```python
from build123d import *

# Parameters (mm, degrees)
SKETCH_1_W          = 19
SKETCH_1_H          = 15
SKETCH_1_R          = 1.1
EXTRUDE_1_DEPTH     = 1.5
SKETCH_1_4_R        = 2.4
EXTRUDE_2_DEPTH     = 14
SKETCH_1_5_R        = 2.85
EXTRUDE_3_DEPTH     = 5.86
SKETCH_1_7_R        = 2.85
CUT_EXTRUDE_1_DEPTH = 4.86
SKETCH_1_8_W        = 0.5
SKETCH_1_8_H        = 0.5
EXTRUDE_4_DEPTH     = 4.86
FILLET_3_SIZE       = 1.5
FILLET_3_SIZE_2     = 2
SKETCH_1_9_W        = 2.5
SKETCH_1_9_H        = 10
EXTRUDE_5_DEPTH     = 4.6


with BuildPart() as part:
    # Sketch 1 → Extrude 1 (new body)
    with BuildSketch(Plane(origin=(0, 0, 0), x_dir=(1, 0, 0), z_dir=(0, 1, 0))):
        with Locations((9.5, 7.5)):
            Rectangle(SKETCH_1_W, SKETCH_1_H)
        with Locations(Location((17, 13, 0), (0, 0, 270))):
            Circle(SKETCH_1_R, mode=Mode.SUBTRACT)
        with Locations(Location((17, 2, 0), (0, 0, 270))):
            Circle(SKETCH_1_R, mode=Mode.SUBTRACT)
    extrude(amount=-EXTRUDE_1_DEPTH)

    # Sketch 1_4 → Extrude 2 (add)
    with BuildSketch(Plane(origin=(0, 0, 0), x_dir=(1, 0, 0), z_dir=(0, 1, 0))):
        with Locations(Location((10, 7.5, 0), (0, 0, 270))):
            Circle(SKETCH_1_4_R)
    extrude(amount=EXTRUDE_2_DEPTH)

    # Sketch 1_5 → Extrude 3 (add)
    with BuildSketch(Plane(origin=(0, 0, 0), x_dir=(1, 0, 0), z_dir=(0, 1, 0))):
        with Locations(Location((10, 7.5, 0), (0, 0, 90))):
            Circle(SKETCH_1_5_R)
    extrude(amount=EXTRUDE_3_DEPTH)

    # Sketch 1_7 → Cut-Extrude 1 (cut)
    with BuildSketch(Plane(origin=(0, 0, 0), x_dir=(1, 0, 0), z_dir=(0, 1, 0))):
        with Locations(Location((10, 7.5, 0), (0, 0, 90))):
            Circle(SKETCH_1_7_R)
    extrude(amount=CUT_EXTRUDE_1_DEPTH, mode=Mode.SUBTRACT)


with BuildPart() as cut_extrude_1_piece_1:
    # of the separate pieces the step leaves, piece 1, a body of its own (cut_extrude_1_pieces)
    add(part.part.solids().sort_by_distance((0, 0, 0))[0])



with BuildPart() as cut_extrude_1_piece_2:
    # of the separate pieces the step leaves, piece 2, a body of its own (cut_extrude_1_pieces)
    add(part.part.solids().sort_by_distance((10, 4.86, -10.35))[0])


with BuildPart() as cut_extrude_1_piece_1_1:
    add(cut_extrude_1_piece_1.part)

    add(cut_extrude_1_piece_2.part)  # Extrude 4 merges Cut-Extrude 1 piece 2
    # Sketch 1_8 → Extrude 4 (add)
    with BuildSketch(Plane(origin=(0, 0, 0), x_dir=(1, 0, 0), z_dir=(0, 1, 0))):
        with Locations((9.262196887, 8.297981086)):
            Rectangle(SKETCH_1_8_W, SKETCH_1_8_H)
        with Locations((9.191679648, 6.064699679)):
            Rectangle(SKETCH_1_8_W, SKETCH_1_8_H)
        with Locations((10.845962172, 6.664377094)):
            Rectangle(SKETCH_1_8_W, SKETCH_1_8_H)
        with Locations((10.845962172, 8.732230249)):
            Rectangle(SKETCH_1_8_W, SKETCH_1_8_H)
    extrude(amount=EXTRUDE_4_DEPTH)

    # Fillet 3
    # an asymmetric fillet: 2, 1.5 mm, written as the material it takes off along each edge
    with BuildSketch(Plane(origin=(10, 14, -7.5), x_dir=(0, 0, 1), z_dir=(-1, 0, 0))) as fillet_3_piece_1:
        with BuildLine():
            Bezier((2.4, -FILLET_3_SIZE), (2.4, 0), (2.4 - FILLET_3_SIZE_2, 0), weights=[1, 0.707106781, 1])
            Line((2.4 - FILLET_3_SIZE_2, 0), (2.4, 0))
            Line((2.4, 0), (2.4, -FILLET_3_SIZE))
        make_face()
    revolve(axis=Axis((10, 14, -7.5), (0, 1, 0)), mode=Mode.SUBTRACT)

    # Sketch 1_9 → Extrude 5 (add)
    with BuildSketch(Plane(origin=(0, 0, 0), x_dir=(1, 0, 0), z_dir=(0, 1, 0))):
        with Locations((2.25, 7.5)):
            Rectangle(SKETCH_1_9_W, SKETCH_1_9_H)
    extrude(amount=EXTRUDE_5_DEPTH)


solid = cut_extrude_1_piece_1_1.part
```
Geometry check sheet. Reference: the model listing, model coordinates, mm. A direction names the side the tool comes from. Coordinates: 2 decimals unless noted, no trailing zeros. Order: outer loops, then holes, each group sorted by start corner. A loop starts at its lowest first (then second) coordinate and runs counter-clockwise, first axis right, second up. Notation, with made-up numbers: M -15,87 L -3,87 A23 cw -3,123 Z; hole C -37,-26.5 d4. An arc over 180 degrees is marked long. One line per question, with ' | ' between items. Start each with the question number.
Item 1: Cross-section at C-C on x = 17. Enter the section's corners in (y, z).
Item 2: Set-up check for faces 1 (the flat face through (2, 2, -2.5)), 2 (the flat face through (11, 5.86, -5)), 3 (the flat face through (2, 2, -12.5)): record each of +Z, -Z, +X, -X, +Y, -Y from which the full face is reachable in a straight line by a thin tool's end or side.
Item 3: Cross-section at B-B on z = -13. Enter the section's corners in (x, y), then the cut area to 3 significant figures.
Item 4: Cross-section at D-D on x = 3.25. Enter the section's corners in (y, z), then the cut area to 3 significant figures.
Item 5: Cross-section at A-A on y = 2.75. Enter the section's corners in (x, z).
Item 6: Draft check along X on faces 4 (the cylindrical face through (15.926, -0.74, -2.238)), 5 (the flat face through (19, -1, -7)), 6 (the flat face through (9, -1, 0)). Enter one of: pulls with the +X half, pulls with the -X half, needs draft (parallel to the pull), parting line crosses it, or undercut.
Item 7: Gauge pin test, flat ends, axial feed: pin 1 (2 mm diameter, centred on x = 17, z = -2, fed in from +Y) (3 decimals); pin 2 (2 mm diameter, centred on x = 6, z = -2.5, fed in from +Y); pin 3 (0.8 mm diameter, centred on x = 3, z = -6.5, fed in from +Y); pin 4 (0.6 mm diameter, centred on y = 3, z = -6.5, fed in from +X). Record the tip position at first contact, or that the pin passes through.
Item 8: Material ranges on L1, parallel to X at y = -1.1, z = -2; L2, parallel to Y at x = 3, z = -5; L3, parallel to Y at x = 7.25, z = -1, recorded low to high. Write a range as [from, to].
Findings:
1) outline: M -1.5,-15 L 0,-15 L 0,-14.1 L -1.5,-14.1 Z; M -1.5,-11.9 L 0,-11.9 L 0,-3.1 L -1.5,-3.1 Z; M -1.5,-0.9 L 0,-0.9 L 0,0 L -1.5,0 Z
2) face 1: +Z, +X, -X, +Y | face 2: +Y | face 3: -Z, +X, -X, +Y
3) outline: M 0,-1.5 L 15.9,-1.5 L 15.9,0 L 0,0 Z; M 18.1,-1.5 L 19,-1.5 L 19,0 L 18.1,0 Z | area: 25.2 mm²
4) outline: M -1.5,-15 L 0,-15 L 0,-12.5 L 4.6,-12.5 L 4.6,-2.5 L 0,-2.5 L 0,0 L -1.5,0 Z | area: 68.5 mm²
5) outline: M 1,-12.5 L 3.5,-12.5 L 3.5,-2.5 L 1,-2.5 Z; M 8.94,-6.31 L 9.44,-6.31 L 9.44,-5.81 L 8.94,-5.81 Z; M 9.01,-8.55 L 9.51,-8.55 L 9.51,-8.05 L 9.01,-8.05 Z; M 10.6,-8.98 L 11.1,-8.98 L 11.1,-8.48 L 10.6,-8.48 Z; M 10.6,-6.91 L 11.1,-6.91 L 11.1,-6.41 L 10.6,-6.41 Z
6) face 4: undercut | face 5: pulls with the +X half | face 6: needs draft
7) pin 1: passes through | pin 2: stops at y = 0 | pin 3: stops at y = 4.6 | pin 4: stops at x = 11.1
8) L1: x = [0, 15.9], [18.1, 19] | L2: y = [-1.5, 4.6] | L3: y = [-1.5, 0]
